Geometry: final body of the model. Coordinates: model frame, mm. A direction names the side the tool comes from. Coordinates: 2 decimals unless noted, no trailing zeros. Order: outer loops, then holes, each group sorted by start corner. A loop starts at its lowest first (then second) coordinate and runs counter-clockwise, first axis right, second up. Notation, with made-up numbers: M -9,81.5 L 3,81.5 A8 cw 3,86.5 Z; hole C 89,17 d2. An arc over 180 degrees is marked long. Write item = value, one per line.
from build123d import *

# Parameters (mm, degrees)
BOX_W             = 134
BOX_H             = 73
BOX_DEPTH         = 25
BOX001_W          = 126
BOX001_H          = 69
BOX001_DEPTH      = 23
BOX002_W          = 10
BOX002_H          = 55
BOX002_DEPTH      = 23
BOX003_W          = 100
BOX003_H          = 30
BOX003_DEPTH      = 1
CYLINDER_R        = 1
CYLINDER_DEPTH    = 5
CYLINDER001_R     = 1
CYLINDER001_DEPTH = 5
CYLINDER002_R     = 3
CYLINDER002_DEPTH = 7
CYLINDER003_R     = 1.5
CYLINDER003_DEPTH = 6
CYLINDER004_R     = 3
CYLINDER004_DEPTH = 7
CYLINDER005_R     = 1.5
CYLINDER005_DEPTH = 6
BOX004_W          = 7
BOX004_H          = 5
BOX004_DEPTH      = 7
BOX005_W          = 7
BOX005_H          = 5
BOX005_DEPTH      = 5
BOX006_W          = 50
BOX006_H          = 20
BOX006_DEPTH      = 4
BOX007_W          = 4
BOX007_H          = 10
BOX007_DEPTH      = 2
CYLINDER006_R     = 1.5
CYLINDER006_DEPTH = 5
CYLINDER007_R     = 1.5
CYLINDER007_DEPTH = 5
BOX008_W          = 5
BOX008_H          = 5
BOX008_DEPTH      = 10
BOX009_W          = 5
BOX009_H          = 5
BOX009_DEPTH      = 10
CYLINDER008_R     = 1.5
CYLINDER008_DEPTH = 5
CYLINDER009_R     = 1.5
CYLINDER009_DEPTH = 5


with BuildPart() as part:
    # Box → Box (join)
    with BuildSketch(Plane.XY):
        with Locations((67, 36.5)):
            Rectangle(BOX_W, BOX_H)
    extrude(amount=BOX_DEPTH)

    # Box001 → Box001 (cut)
    with BuildSketch(Plane(origin=(6, 2, 2), x_dir=(1, 0, 0), z_dir=(0, 0, 1))):
        with Locations((63, 34.5)):
            Rectangle(BOX001_W, BOX001_H)
    extrude(amount=BOX001_DEPTH, mode=Mode.SUBTRACT)

    # Box002 → Box002 (cut)
    with BuildSketch(Plane(origin=(-2, 7, 2), x_dir=(1, 0, 0), z_dir=(0, 0, 1))):
        with Locations((5, 27.5)):
            Rectangle(BOX002_W, BOX002_H)
    extrude(amount=BOX002_DEPTH, mode=Mode.SUBTRACT)

    # Box003 → Box003 (cut)
    with BuildSketch(Plane(origin=(31, 35, 1), x_dir=(1, 0, 0), z_dir=(0, 0, 1))):
        with Locations((50, 15)):
            Rectangle(BOX003_W, BOX003_H)
    extrude(amount=BOX003_DEPTH, mode=Mode.SUBTRACT)

    # Cylinder → Cylinder (join)
    with BuildSketch(Plane(origin=(129, 37, 1), x_dir=(1, 0, 0), z_dir=(0, 0, 1))):
        Circle(CYLINDER_R)
    extrude(amount=CYLINDER_DEPTH)

    # Cylinder001 → Cylinder001 (join)
    with BuildSketch(Plane(origin=(129, 63, 1), x_dir=(1, 0, 0), z_dir=(0, 0, 1))):
        Circle(CYLINDER001_R)
    extrude(amount=CYLINDER001_DEPTH)

    # Cylinder002 → Cylinder002 (join)
    with BuildSketch(Plane(origin=(114, 31, 1), x_dir=(1, 0, 0), z_dir=(0, 0, 1))):
        Circle(CYLINDER002_R)
    extrude(amount=CYLINDER002_DEPTH)

    # Cylinder003 → Cylinder003 (cut)
    with BuildSketch(Plane(origin=(114, 31, 3), x_dir=(1, 0, 0), z_dir=(0, 0, 1))):
        Circle(CYLINDER003_R)
    extrude(amount=CYLINDER003_DEPTH, mode=Mode.SUBTRACT)

    # Cylinder004 → Cylinder004 (join)
    with BuildSketch(Plane(origin=(56, 31, 2), x_dir=(1, 0, 0), z_dir=(0, 0, 1))):
        Circle(CYLINDER004_R)
    extrude(amount=CYLINDER004_DEPTH)

    # Cylinder005 → Cylinder005 (cut)
    with BuildSketch(Plane(origin=(56, 31, 3), x_dir=(1, 0, 0), z_dir=(0, 0, 1))):
        Circle(CYLINDER005_R)
    extrude(amount=CYLINDER005_DEPTH, mode=Mode.SUBTRACT)

    # Box004 → Box004 (cut)
    with BuildSketch(Plane(origin=(61, 74, 8), x_dir=(1, 0, 0), z_dir=(0, -1, 0))):
        with Locations((3.5, 2.5)):
            Rectangle(BOX004_W, BOX004_H)
    extrude(amount=BOX004_DEPTH, mode=Mode.SUBTRACT)

    # Box005 → Box005 (cut)
    with BuildSketch(Plane(origin=(61, 74, 15), x_dir=(1, 0, 0), z_dir=(0, -1, 0))):
        with Locations((3.5, 2.5)):
            Rectangle(BOX005_W, BOX005_H)
    extrude(amount=BOX005_DEPTH, mode=Mode.SUBTRACT)

    # Box006 → Box006 (join)
    with BuildSketch(Plane(origin=(76, 71, 2), x_dir=(1, 0, 0), z_dir=(0, -1, 0))):
        with Locations((25, 10)):
            Rectangle(BOX006_W, BOX006_H)
    extrude(amount=BOX006_DEPTH)

    # Box007 → Box007 (cut)
    with BuildSketch(Plane(origin=(134, 41.5, 25), x_dir=(0, 0, -1), z_dir=(-1, 0, 0))):
        with Locations((2, 5)):
            Rectangle(BOX007_W, BOX007_H)
    extrude(amount=BOX007_DEPTH, mode=Mode.SUBTRACT)

    # Cylinder006 → Cylinder006 (cut)
    with BuildSketch(Plane(origin=(3, 3.5, 20), x_dir=(0, 1, 0), z_dir=(0, 0, 1))):
        Circle(CYLINDER006_R)
    extrude(amount=CYLINDER006_DEPTH, mode=Mode.SUBTRACT)

    # Cylinder007 → Cylinder007 (cut)
    with BuildSketch(Plane(origin=(3, 69.5, 20), x_dir=(0, 1, 0), z_dir=(0, 0, 1))):
        Circle(CYLINDER007_R)
    extrude(amount=CYLINDER007_DEPTH, mode=Mode.SUBTRACT)

    # Box008 → Box008 (join)
    with BuildSketch(Plane(origin=(132, 2, 15), x_dir=(0, 1, 0), z_dir=(0, 0, 1))):
        with Locations((2.5, 2.5)):
            Rectangle(BOX008_W, BOX008_H)
    extrude(amount=BOX008_DEPTH)

    # Box009 → Box009 (join)
    with BuildSketch(Plane(origin=(132, 66, 15), x_dir=(0, 1, 0), z_dir=(0, 0, 1))):
        with Locations((2.5, 2.5)):
            Rectangle(BOX009_W, BOX009_H)
    extrude(amount=BOX009_DEPTH)

    # Cylinder008 → Cylinder008 (cut)
    with BuildSketch(Plane(origin=(130.5, 69.5, 20), x_dir=(0, 1, 0), z_dir=(0, 0, 1))):
        Circle(CYLINDER008_R)
    extrude(amount=CYLINDER008_DEPTH, mode=Mode.SUBTRACT)

    # Cylinder009 → Cylinder009 (cut)
    with BuildSketch(Plane(origin=(130.5, 3.5, 20), x_dir=(0, 1, 0), z_dir=(0, 0, 1))):
        Circle(CYLINDER009_R)
    extrude(amount=CYLINDER009_DEPTH, mode=Mode.SUBTRACT)


solid = part.part
1) Mould query, pull axis X, two halves, no side actions, for faces 4 (the face through (130, 69, 20)), 5 (the face through (3, 7, 13)), 6 (the face through (134, 36, 12)). Classes: pulls with the +X half, pulls with the -X half, needs draft (parallel to the pull), parting line crosses it, or undercut.
Numbers:
face_4 = undercut
face_5 = needs draft
face_6 = pulls with the +X half
2) Section D-D, the plane y = 69.5. Return loops of the section in (x, z), and give its area (3 significant figures).
Numbers:
outline = M 0,0 L 134,0 L 134,25 L 132,25 L 132,20 L 129,20 L 129,25 L 127,25 L 127,15 L 132,15 L 132,2 L 126,2 L 126,22 L 76,22 L 76,2 L 6,2 L 6,25 L 4.5,25 L 4.5,20 L 1.5,20 L 1.5,25 L 0,25 Z
area = 1,470 mm²
3) Section B-B, the plane y = 56.5. Return loops of the section in (x, z).
Numbers:
outline = M 0,0 L 134,0 L 134,25 L 132,25 L 132,2 L 131,2 L 131,1 L 31,1 L 31,2 L 0,2 Z
4) Section C-C, the plane x = 114. Return loops of the section in (y, z), and give its area (3 significant figures).
Numbers:
outline = M 0,0 L 73,0 L 73,25 L 71,25 L 71,22 L 67,22 L 67,2 L 65,2 L 65,1 L 35,1 L 35,2 L 34,2 L 34,8 L 32.5,8 L 32.5,3 L 29.5,3 L 29.5,8 L 28,8 L 28,2 L 2,2 L 2,25 L 0,25 Z
area = 309 mm²
5) Set-up query: faces 1 (the face through (129.013, 3.305, 22.465)), 2 (the face through (129, 4, 15)), 3 (the face through (0, 42, 1)). Return all of +Z, -Z, +X, -X, +Y, -Y with unobstructed straight access to the full face (end or side cutting, diameter ignored); none if empty.
Numbers:
face_1 = +Z
face_2 = none
face_3 = +Z, -Z, -X, +Y, -Y
6) Pin query (flat end, axial travel): pin 1 (3.5 mm diameter, centred on x = 3.5, y = 3, fed in from +Z); pin 2 (4 mm diameter, centred on y = 35, z = 18.5, fed in from -X); pin 3 (5 mm diameter, centred on x = 56, y = 31, fed in from +Z); pin 4 (0.9 mm diameter, centred on x = 113.5, y = 31.5, fed in from +Z). Return the tip coordinate at first contact, or that it passes through.
Numbers:
pin_1 = 25
pin_2 = 132
pin_3 = 9
pin_4 = 3
7) Line query: L1, parallel to X at y = 3.5, z = 22.4; L2, parallel to Y at x = 130.5, z = 23.6; L3, parallel to Y at x = 56, z = 7.15. Output: solid intervals per line, ascending.
Numbers:
L1 = 0 to 1.5, 4.5 to 6, 127 to 129, 132 to 134
L2 = 0 to 2, 5 to 7, 66 to 68, 71 to 73
L3 = 0 to 2, 28 to 29.5, 32.5 to 34, 71 to 73
8) Section A-A, the plane x = 56. Return loops of the section in (y, z).
Numbers:
outline = M 0,0 L 73,0 L 73,25 L 71,25 L 71,2 L 65,2 L 65,1 L 35,1 L 35,2 L 34,2 L 34,9 L 32.5,9 L 32.5,3 L 29.5,3 L 29.5,9 L 28,9 L 28,2 L 2,2 L 2,25 L 0,25 Z
